Part model, mm, in its own coordinate system. Face numbers are marked on the shaded views. A direction names the side the tool comes from. Round coordinates to 2 decimals unless told otherwise and drop trailing zeros. Loops run counter-clockwise (first coordinate to the right, second up) from the corner with the lowest first, then second, coordinate; pieces in that order, holes last. Notation, with made-up numbers: (18, 22) -> (28, 22) arc R23 ccw to (28, 44) -> close; hole circle Ø7 at (-1, 84). An arc over 180 degrees is marked (long way). Answer as CSV lines item,"result".
Autodesk Inventor part; units mm, degrees
ref_plane "YZ Plane" through (0, 0, 0) normal (1, 0, 0) x (0, 1, 0)
ref_plane "XZ Plane" through (0, 0, 0) normal (0, 1, 0) x (-1, 0, 0)
ref_plane "XY Plane" through (0, 0, 0) normal (0, 0, 1) x (1, 0, 0)
sketch "Sketch1" plane through (0, 0, 0) normal (0, 0, 1) x (1, 0, 0)
  line L0 (0, 0) -> (6, 0)
  line L1 (6, 0) -> (6, 2)
  line L2 (6, 2) -> (0, 2)
  line L3 (0, 2) -> (0, 0)
  dimension "d0" = 6
  dimension "d1" = 2
extrude "Extrusion1" add sketch "Sketch1" along normal blind 5
sketch "Sketch2" plane through (0, 0, 0) normal (-1, 0, 0) x (0, 0, 1)
  line L0 (0, 2) -> (0, 0)
  line L1 (0, 0) -> (5, 0)
  line L2 (5, 2) -> (5, 0)
  line L3 (0, 2) -> (5, 2)
extrude "Extrusion2" add sketch "Sketch2" along normal blind 2
sketch "Sketch3" plane through (6, 0, 0) normal (0, -1, 0) x (1, 0, 0)
  line L0 (-8, 5) -> (-6, 5)
  line L1 (-6, 5) -> (-6, 0)
  line L2 (-6, 0) -> (-8, 0)
  line L3 (-8, 0) -> (-8, 5)
extrude "Extrusion3" add sketch "Sketch3" along normal blind 10.5
sketch "Sketch5" plane through (6, 0, 0) normal (0, -1, 0) x (1, 0, 0)
  line L0 (0, 5) -> (-8, 5)
  line L1 (0, 0) -> (-8, 0)
  line L2 (0, 5) -> (-2, 5)
  line L3 (-2, 5) -> (-2, 0)
  line L4 (-2, 0) -> (0, 0)
  line L5 (0, 0) -> (0, 5)
extrude "Extrusion5" add sketch "Sketch5" along normal blind 4
sketch "Sketch6" plane through (6, 2, 5) normal (1, 0, 0) x (0, 0, -1)
  line L0 (0, -6) -> (5, -6)
  line L1 (5, -2) -> (5, -12.5)
  line L2 (0, -6) -> (5, -6)
  line L3 (5, -6) -> (5, -4)
  line L4 (5, -4) -> (0, -4)
  line L5 (0, -4) -> (0, -6)
  dimension "d13" = 2
extrude "Extrusion6" add sketch "Sketch6" along normal blind 89.93
sketch "Sketch7" plane through (95.93, 2, 5) normal (1, 0, 0) x (0, 0, -1)
  line L0 (0, -6) -> (5, -6)
  line L1 (5, -6) -> (5, -4)
  line L2 (5, -4) -> (0, -4)
  line L3 (0, -4) -> (0, -6)
  point P0 (5, -2)
extrude "Extrusion7" add sketch "Sketch7" along normal blind 2
sketch "Sketch8" plane through (6, -4, 0) normal (0, -1, 0) x (1, 0, 0)
  line L0 (-2, 0) -> (91.93, 0)
  line L1 (91.93, 5) -> (89.93, 5)
  line L2 (89.93, 5) -> (89.93, 0)
  line L3 (89.93, 0) -> (91.93, 0)
  line L4 (91.93, 0) -> (91.93, 5)
  point P0 (-6, 0)
  dimension "d18" = 2
extrude "Extrusion8" add sketch "Sketch8" along normal blind 10
sketch "Sketch9" plane through (6, -10.5, 0) normal (0, -1, 0) x (1, 0, 0)
  line L0 (-6, 0) -> (-6, 5)
  line L1 (-6, 5) -> (-8, 5)
  line L2 (-8, 5) -> (-8, 0)
  line L3 (-8, 0) -> (-6, 0)
extrude "Extrusion9" add sketch "Sketch9" along normal blind 5
sketch "Sketch10" plane through (0, 0, 5) normal (1, 0, 0) x (0, 0, -1)
  line L0 (0, 2) -> (0, -15.5)
  line L1 (5, 2) -> (5, -15.5)
  line L2 (0, -15.5) -> (5, -15.5)
  line L3 (5, -15.5) -> (5, -13.5)
  line L4 (5, -13.5) -> (0, -13.5)
  line L5 (0, -13.5) -> (0, -15.5)
  dimension "d23" = 2
extrude "Extrusion10" add sketch "Sketch10" along normal blind 5
sketch "Sketch11" plane through (5, 0, 5) normal (1, 0, 0) x (0, 0, -1)
  line L0 (0, -15.5) -> (5, -15.5)
  line L1 (5, -15.5) -> (5, -13.5)
  line L2 (5, -13.5) -> (0, -13.5)
  line L3 (0, -13.5) -> (0, -15.5)
  point P0 (5, 0)
extrude "Extrusion11" add sketch "Sketch11" along normal blind 2
sketch "Sketch12" plane through (0, -13.5, 5) normal (0, 1, 0) x (1, 0, 0)
  line L0 (0, 0) -> (7, 0)
  line L1 (7, 5) -> (5, 5)
  line L2 (5, 5) -> (5, 0)
  line L3 (5, 0) -> (7, 0)
  line L4 (7, 0) -> (7, 5)
  dimension "d28" = 2
extrude "Extrusion12" add sketch "Sketch12" along normal blind 2
sketch "Sketch13" plane through (95.93, -4, 0) normal (-1, 0, 0) x (0, 0, 1)
  line L0 (5, 0) -> (5, -10)
  line L1 (0, -10) -> (5, -10)
  line L2 (5, -10) -> (5, -8)
  line L3 (5, -8) -> (0, -8)
  line L4 (0, -8) -> (0, -10)
  point P0 (0, 4)
  dimension "d31" = 2
extrude "Extrusion13" add sketch "Sketch13" along normal blind 5
sketch "Sketch14" plane through (0, 0, 5) normal (0, 0, 1) x (1, 0, 0)
  line L0 (97.93, -14) -> (90.93, -14)
  line L1 (90.93, -12) -> (92.93, -12)
  line L2 (92.93, -12) -> (92.93, -14)
  line L3 (92.93, -14) -> (90.93, -14)
  line L4 (90.93, -14) -> (90.93, -12)
  dimension "d34" = 2
extrude "Extrusion14" add sketch "Sketch14" along normal blind 5
sketch "Sketch15" plane through (92.93, -14, 5) normal (1, 0, 0) x (0, 0, -1)
  line L0 (0, 0) -> (-5, 0)
  line L1 (-5, 2) -> (-3, 2)
  line L2 (-3, 2) -> (-3, 0)
  line L3 (-3, 0) -> (-5, 0)
  line L4 (-5, 0) -> (-5, 2)
  point P0 (5, 14)
  dimension "d37" = 2
extrude "Extrusion15" add sketch "Sketch15" along normal blind 4
sketch "Sketch16" plane through (0, 0, 10) normal (0, 0, 1) x (1, 0, 0)
  line L0 (90.93, -12) -> (90.93, -14)
  line L1 (90.93, -14) -> (96.93, -14)
  line L2 (95.93, -12) -> (90.93, -12)
  line L3 (97.93, -14) -> (92.93, -14)
  line L4 (90.93, -12) -> (92.93, -12)
  line L5 (92.93, -12) -> (92.93, -14)
  line L6 (92.93, -14) -> (90.93, -14)
  line L7 (90.93, -14) -> (90.93, -12)
  point P0 (0, 0)
extrude "Extrusion16" add sketch "Sketch16" along normal blind 5
sketch "Sketch17" plane through (92.93, -14, 10) normal (1, 0, 0) x (0, 0, -1)
  line L0 (-5, 2) -> (-5, 0)
  line L1 (10, 0) -> (-5, 0)
  line L2 (-5, 2) -> (-3, 2)
  line L3 (-3, 2) -> (-3, 0)
  line L4 (-3, 0) -> (-5, 0)
  line L5 (-5, 0) -> (-5, 2)
  point P0 (10, 14)
  dimension "d42" = 2
extrude "Extrusion17" add sketch "Sketch17" along normal blind 4
sketch "Sketch18" plane through (0, 0, 15) normal (0, 0, 1) x (1, 0, 0)
  line L0 (90.93, -12) -> (90.93, -14)
  line L1 (90.93, -12) -> (90.93, -14)
  line L2 (97.93, -14) -> (90.93, -14)
  line L3 (90.93, -12) -> (92.93, -12)
  line L4 (92.93, -12) -> (92.93, -14)
  line L5 (92.93, -14) -> (90.93, -14)
  line L6 (90.93, -14) -> (90.93, -12)
  point P0 (0, 0)
  dimension "d45" = 2
extrude "Extrusion18" add sketch "Sketch18" along normal blind 10
sketch "Sketch19" plane through (92.93, -14, 15) normal (1, 0, 0) x (0, 0, -1)
  line L0 (15, 2) -> (-10, 2)
  line L1 (15, 0) -> (-10, 0)
  line L2 (-3, 2) -> (-5, 2)
  line L3 (-5, 2) -> (-5, 0)
  line L4 (-5, 0) -> (-3, 0)
  line L5 (-3, 0) -> (-3, 2)
  line L6 (0, 2) -> (0, 0)
  point P0 (15, 14)
  dimension "d48" = 2
  dimension "d51" = 3
extrude "Extrusion19" add sketch "Sketch19" along normal blind 4 contours L5 L1 L3 L0
sketch "Sketch20" plane through (92.93, -14, 25) normal (1, 0, 0) x (0, 0, -1)
  line L0 (25, 2) -> (0, 2)
  line L1 (25, 0) -> (0, 0)
  line L2 (0, 2) -> (2, 2)
  line L3 (2, 2) -> (2, 0)
  line L4 (2, 0) -> (0, 0)
  line L5 (0, 0) -> (0, 2)
  point P0 (25, 14)
  dimension "d52" = 2
extrude "Extrusion20" add sketch "Sketch20" along normal blind 4
properties part number "Steunbalk boven"
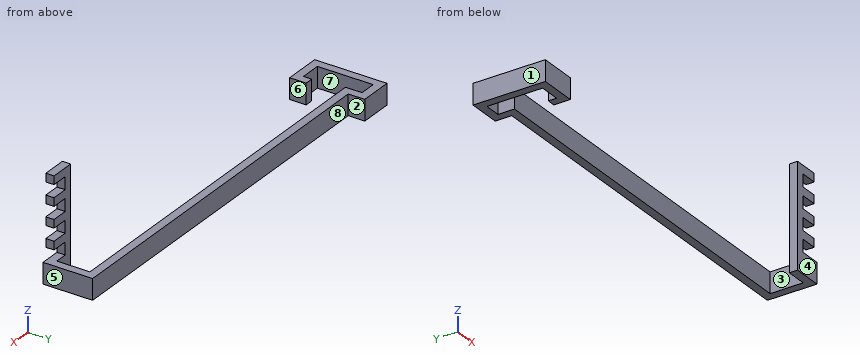
Q1. Saw through at D-D, the plane z = 21.25. Write the cut outline in (x, y), then the cut area to 3 significant figures.
Geometry results:
outline,"(90.93, -14) -> (92.93, -14) -> (92.93, -12) -> (90.93, -12) -> close"
area,"4.00 mm2"
Q2. Two-plate mould, pull along Y, no slides. Class the marked faces 6, 7 and 8: pulls with the +Y half, pulls with the -Y half, needs draft (parallel to the pull), parting line crosses it, or undercut.
Geometry results:
face 6,"needs draft"
face 7,"undercut"
face 8,"pulls with the +Y half"
Q3. Saw through at A-A, the plane y = -3. Write the cut outline in (x, z), then the cut area to 3 significant figures.
Geometry results:
outline,"(-2, 0) -> (0, 0) -> (0, 5) -> (-2, 5) -> close; (4, 0) -> (97.93, 0) -> (97.93, 5) -> (4, 5) -> close"
area,"480 mm2"
Q4. Saw through at B-B, the plane z = 2.5. Write the cut outline in (x, y), then the cut area to 3 significant figures.
Geometry results:
outline,"(-2, -15.5) -> (7, -15.5) -> (7, -11.5) -> (5, -11.5) -> (5, -13.5) -> (0, -13.5) -> (0, 0) -> (4, 0) -> (4, -4) -> (95.93, -4) -> (95.93, -12) -> (90.93, -12) -> (90.93, -14) -> (97.93, -14) -> (97.93, -2) -> (6, -2) -> (6, 2) -> (-2, 2) -> close"
area,"287 mm2"
Q5. Saw through at C-C, the plane x = 19. Write the cut outline in (y, z), then the cut area to 3 significant figures.
Geometry results:
outline,"(-4, 0) -> (-2, 0) -> (-2, 5) -> (-4, 5) -> close"
area,"10.0 mm2"
Q6. Drop flat-ended pins along their axis: P1, Ø0.6, axis at y = -12.5, z = 19, coming from the +X side; P2, Ø0.6, axis at y = -12.5, z = 17, coming from the +X side; P3, Ø5.5, axis at x = 93.5, z = 10, coming from the -Y side. Give the stop position or say it passes through.
Geometry results:
P1,"x = 96.93"
P2,"x = 92.93"
P3,"y = -14"
Q7. Drill centre lines: line 1 along X through (y, z) = (-5.5, 4.5); line 2 along Y through (x, z) = (3, 4.5); line 3 along Y through (x, z) = (72, 1.5). Where is each one in solid material? Low to high.
Geometry results:
line 1,"-2 to 0, 95.93 to 97.93"
line 2,"-15.5 to -13.5, 0 to 2"
line 3,"-4 to -2"
Q8. Which spindle directions (+Z, -Z, +X, -X, +Y, -Y) get a long thin tool onto all of the face, cutting with end or side? Do the marked faces 1, 2, 3, 4 and 5. Say none if no direction does.
Geometry results:
face 1,"+Z, -Z, -X, +Y, -Y"
face 2,"+Z, -Z, +X, +Y"
face 3,"+Z, -Z"
face 4,"+Z, -Z, +X, -Y"
face 5,"+Z, -Z, +X, +Y, -Y"
